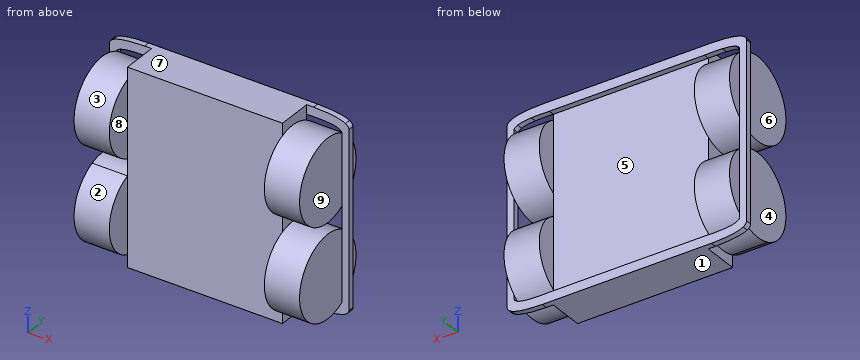
Autodesk Inventor part; units mm, degrees
ref_plane "YZ Plane" through (0, 0, 0) normal (1, 0, 0) x (0, 1, 0)
ref_plane "XZ Plane" through (0, 0, 0) normal (0, 1, 0) x (-1, 0, 0)
ref_plane "XY Plane" through (0, 0, 0) normal (0, 0, 1) x (1, 0, 0)
sketch "Эскиз1" plane through (0, 0, 0) normal (0, 1, 0) x (-1, 0, 0)
  line L0 (0, 0) -> (-132, 0)
  line L1 (-132, 0) -> (-132, -165.5)
  line L2 (-132, -165.5) -> (0, -165.5)
  line L3 (0, -165.5) -> (0, 0)
  line L4 (0, 0) -> (-132, 0)
  line L5 (-132, 0) -> (-132, -8)
  line L6 (-132, -8) -> (0, -8)
  line L7 (0, -8) -> (0, 0)
  line L8 (0, -165.5) -> (-132, -165.5)
  line L9 (-132, -165.5) -> (-132, -157.5)
  line L10 (-132, -157.5) -> (0, -157.5)
  line L11 (0, -157.5) -> (0, -165.5)
  line L12 (0, 0) -> (0, -43)
  line L13 (0, -43) -> (0, -8)
  line L14 (0, -8) -> (30, -8)
  line L15 (30, -8) -> (30, -78)
  line L16 (30, -78) -> (0, -78)
  line L17 (0, -78) -> (0, -8)
  line L18 (0, -157.5) -> (30, -157.5)
  line L19 (30, -157.5) -> (30, -87.5)
  line L20 (30, -87.5) -> (0, -87.5)
  line L21 (0, -87.5) -> (0, -157.5)
  line L22 (-132, -8) -> (-162, -8)
  line L23 (-162, -8) -> (-162, -78)
  line L24 (-162, -78) -> (-132, -78)
  line L25 (-132, -78) -> (-132, -8)
  line L26 (-132, -157.5) -> (-162, -157.5)
  line L27 (-162, -157.5) -> (-162, -87.5)
  line L28 (-162, -87.5) -> (-132, -87.5)
  line L29 (-132, -87.5) -> (-132, -157.5)
  dimension "d0" = 132
  dimension "d1" = 165.5
  dimension "d2" = 8
  dimension "d3" = 8
  dimension "d4" = 43
  dimension "d5" = 35
  dimension "d6" = 30
  dimension "d7" = 70
  dimension "d8" = 30
  dimension "d9" = 70
  dimension "d10" = 30
  dimension "d11" = 70
  dimension "d12" = 30
  dimension "d13" = 70
extrude "Выдавливание1" add sketch "Эскиз1" along normal blind 30 contours L3 L6 L1 L0 | L3 L10 L1 L6 | L10 L3 L2 L1
sketch "Эскиз2" plane through (132, 0, 0) normal (1, 0, 0) x (0, 0, -1)
  line L0 (0, 0) -> (0, 30)
  line L1 (165.5, 0) -> (165.5, 30)
  line L2 (165.5, 0) -> (0, 0)
  line L3 (0, 0) -> (43, 0)
  line L4 (43, 0) -> (43, 4.5763)
  line L5 (43, 4.5763) -> (43, 30)
  line L6 (43, 0) -> (43, 12.5)
  line L7 (165.5, 0) -> (122.5, 0)
  line L8 (122.5, 0) -> (122.5, 12.5)
  line L9 (122.5, 12.5) -> (43, 12.5)
  circle A0 centre (43, 12.5) radius 35
  circle A1 centre (122.5, 12.5) radius 35
  dimension "d24" = 43
  dimension "d25" = 12.5
  dimension "d26" = 43
  dimension "d27" = 70
  dimension "d28" = 70
extrude "Выдавливание2" add sketch "Эскиз2" along normal blind 30 contours A1 L2 | L2 L8 L9 A1 | L2 A1 L9 L8 | A0 L2 | L2 L4 L5 L9 A0 | L2 A0 L9 L5 L4
sketch "Эскиз3" plane through (0, 0, -165.5) normal (-1, 0, 0) x (0, 0, 1)
  circle A0 centre (122.5, 12.5) radius 35
  circle A1 centre (122.5, 12.5) radius 35
  arc A2 (10.3083, 0) -> (75.6917, 0) centre (43, 12.5) ccw
  circle A3 centre (43, 12.5) radius 35
  point P0 (165.5, 0)
  point P1 (122.5, 15)
  point P2 (43, 15)
  point P3 (75.6917, 0)
extrude "Выдавливание3" add sketch "Эскиз3" along normal blind 30
sketch "Эскиз4" plane through (0, 30, 0) normal (0, 1, 0) x (1, 0, 0)
  line L0 (-30, 78) -> (-30, 8)
  line L1 (-36, 8) -> (-36, 0)
  line L2 (132, 165.5) -> (0, 165.5)
  line L3 (-36, 0) -> (0, 0)
  line L4 (0, 0) -> (0, 165.5)
  line L5 (0, 165.5) -> (-36, 165.5)
  line L6 (-36, 165.5) -> (-36, 0)
  line L7 (132, 152.8109) -> (132, 165.5)
  line L8 (132, 165.5) -> (168, 165.5)
  line L9 (168, 165.5) -> (168, 0)
  line L10 (168, 0) -> (132, 0)
  line L11 (132, 0) -> (132, 165.5)
  line L12 (0, 8) -> (-30, 8)
  line L13 (-30, 157.5) -> (-30, 87.5)
  line L14 (0, 8) -> (-30, 8)
  line L15 (-30, 8) -> (-30, 157.5)
  line L16 (-30, 157.5) -> (0, 157.5)
  line L17 (0, 157.5) -> (0, 8)
  line L18 (162, 8) -> (162, 78)
  line L19 (132, 157.5) -> (162, 157.5)
  line L20 (162, 157.5) -> (162, 8)
  line L21 (162, 8) -> (132, 8)
  line L22 (132, 8) -> (132, 157.5)
  line L23 (168, 0) -> (-36, 0)
  line L24 (-36, 0) -> (-36, 165.5)
  line L25 (-36, 165.5) -> (168, 165.5)
  line L26 (168, 165.5) -> (168, 0)
  line L27 (0, 157.5) -> (132, 157.5)
  line L28 (132, 157.5) -> (132, 165.5)
  line L29 (132, 165.5) -> (0, 165.5)
  line L30 (0, 165.5) -> (0, 157.5)
  line L31 (0, 8) -> (0, 12.6891)
  line L32 (132, 0) -> (0, 0)
  line L33 (0, 0) -> (0, 8)
  line L34 (0, 8) -> (132, 8)
  line L35 (132, 8) -> (132, 0)
  line L36 (168, 165.5) -> (165, 165.5)
  line L37 (165, 165.5) -> (165, 161.5)
  line L38 (165, 161.5) -> (168, 161.5)
  line L39 (168, 161.5) -> (168, 165.5)
  line L40 (168, 0) -> (165, 0)
  line L41 (165, 0) -> (165, 4)
  line L42 (165, 4) -> (168, 4)
  line L43 (168, 4) -> (168, 0)
  line L44 (-36, 0) -> (-33, 0)
  line L45 (-33, 0) -> (-33, 4)
  line L46 (-33, 4) -> (-36, 4)
  line L47 (-36, 4) -> (-36, 0)
  line L48 (-36, 165.5) -> (-33, 165.5)
  line L49 (-33, 165.5) -> (-33, 161.5)
  line L50 (-33, 161.5) -> (-36, 161.5)
  line L51 (-36, 161.5) -> (-36, 165.5)
  line L52 (0, 165.5) -> (0, 155.1917)
  spline S0 degree 2 poles (0, 165.5) (-35.5316, 165.8812) (-36, 157.5) knots 0 0 0 1 1 1
  spline S1 degree 2 poles (132, 165.5) (167.5316, 165.8812) (168, 157.5) knots 0 0 0 1 1 1
  spline S2 degree 2 poles (132, 0) (167.5316, -0.3812) (168, 8) knots 0 0 0 1 1 1
  line L53 (0, 0) -> (132, 0)
  spline S3 degree 2 poles (0, 0) (-35.5316, -0.3812) (-36, 8) knots 0 0 0 1 1 1
  line L54 (-30, 8) -> (-27, 8)
  line L55 (-27, 8) -> (-27, 10)
  line L56 (-27, 10) -> (-30, 10)
  line L57 (-30, 10) -> (-30, 8)
  spline S4 degree 2 poles (0, 8) (-28.3192, 6.9002) (-30, 12.6891) knots 0 0 0 1 1 1
  line L58 (162, 8) -> (159, 8)
  line L59 (159, 8) -> (159, 10)
  line L60 (159, 10) -> (162, 10)
  line L61 (162, 10) -> (162, 8)
  line L62 (162, 157.5) -> (159, 157.5)
  line L63 (159, 157.5) -> (159, 155.5)
  line L64 (159, 155.5) -> (162, 155.5)
  line L65 (162, 155.5) -> (162, 157.5)
  line L66 (-30, 157.5) -> (-27, 157.5)
  line L67 (-27, 157.5) -> (-27, 155.5)
  line L68 (-27, 155.5) -> (-30, 155.5)
  line L69 (-30, 155.5) -> (-30, 157.5)
  spline S5 degree 2 poles (-30, 152.8109) (-28.3192, 158.5998) (0, 157.5) knots 0 0 0 1 1 1
  line L70 (162, 87.5) -> (162, 157.5)
  spline S6 degree 2 poles (132, 157.5) (160.3192, 158.5998) (162, 152.8109) knots 0 0 0 1 1 1
  spline S7 degree 2 poles (132, 8) (160.3192, 6.9002) (162, 12.6891) knots 0 0 0 1 1 1
  point P0 (0, 10.3083)
  point P1 (162, 152.8109)
  point P2 (137.9176, 0)
  point P3 (168, 8)
  point P4 (168, 157.5)
  point P5 (137.9176, 165.5)
  point P6 (-5.9176, 165.5)
  point P7 (-36, 157.5)
  point P8 (-5.9176, 0)
  point P9 (-30, 12.6891)
  point P10 (-30, 152.8109)
  dimension "d30" = 36
  dimension "d31" = 3
  dimension "d32" = 3
  dimension "d33" = 3
  dimension "d34" = 2
  dimension "d35" = 3
  dimension "d36" = 2
  dimension "d37" = 3
  dimension "d38" = 2
extrude "Выдавливание4" add sketch "Эскиз4" along normal blind 5 contours L0 L12 S4 L4 L3 S3 L6 S0 L5 S5 L16 L13 L15 | S4 L56 L0 | L56 L55 L12 L0 | S4 L12 L55 | L13 L68 S5 | L13 L16 L67 L68 | L67 L16 S5 | L34 L11 L23 L4 | S7 L21 L18 L20 L19 S6 L7 L8 S1 L9 S2 L10 L11 | L4 L2 L7 L27 | S7 L59 L21 | L59 L60 L18 L21 | S7 L18 L60 | L19 L63 S6 | L19 L20 L64 L63 | L64 L20 S6
sketch "Эскиз6" plane through (0, 30, 0) normal (0, 1, 0) x (1, 0, 0)
  line L0 (168, 8) -> (168, 157.5)
  line L1 (-36, 157.5) -> (-36, 8)
  line L2 (162, 16.1905) -> (162, 69.8095)
  line L3 (-30, 69.8095) -> (-30, 16.1905)
  line L4 (132, 12.6891) -> (132, 73.3109)
  line L5 (0, 73.3109) -> (0, 12.6891)
  line L6 (187.3576, 0) -> (377.3576, 0)
  line L7 (377.3576, 0) -> (377.3576, 165.5)
  line L8 (377.3576, 165.5) -> (187.3576, 165.5)
  line L9 (187.3576, 165.5) -> (187.3576, 0)
  point P0 (0, 0)
  dimension "d41" = 204
  dimension "d42" = 192
  dimension "d43" = 132
  dimension "d44" = 190
  dimension "d45" = 165.5
Part model, mm, in its own coordinate system. Face numbers are marked on the shaded views. A direction names the side the tool comes from. Coordinates: 2 decimals unless noted, no trailing zeros. Loops run counter-clockwise (first coordinate to the right, second up) from the corner with the lowest first, then second, coordinate; pieces in that order, holes last. Notation, with made-up numbers: (13, -32) - (58, -32) arc R27 cw to (58, -16) - close; hole circle Ø8 at (-8.75, 47.25). An arc over 180 degrees is marked (long way). Write item = value, one per line. Start each with the question number.
Item 1: 3-axis set-ups, long thin cutter, end or side, ignore diameter. For the marked faces 5, 6, 7, 8 and 9: which of +Z, -Z, +X, -X, +Y, -Y reach the whole face in a straight line?
Item 2: Flat gauge pins, fed straight in: pin 1 Ø10 at (y, z) = (43, -37.5) entering from -X; pin 2 Ø12 at (y, z) = (38.5, -71.5) entering from +X; pin 3 Ø24.5 at (y, z) = (-8.5, -116.5) entering from +X; pin 4 Ø8 at (x, z) = (122.5, -85) entering from -Y. Where does each tip first touch, or does it go through?
Item 3: Cut at D-D, the plane x = 142. State how many separate pieces and enclosed holes the cut face has, and give its area (3 significant figures).
Item 4: Cut at C-C, the plane z = -43. Give the cut face in (x, y).
Item 5: Wall check: L1, parallel to X at y = -10.5, z = -102.5; L2, parallel to Y at x = 122.5, z = -27; L3, parallel to X at y = 10, z = -22. Give the ranges that are in metal, low to high. Write a range as from..to.
Item 6: Mould opens along Z. For the marked faces 1, 2, 3 and 4 say: released by +Z, released by -Z, zero draft, split by the parting line, or undercut.
Item 7: Cut at B-B, the plane x = 96.5. Give the cut face in (y, z).
Item 8: Cut at A-A, the plane y = 12.5. Give the cut face in (x, z).
The answers:
q1.face_5 = +Y
q1.face_6 = +Z, -Z, -X, -Y
q1.face_7 = +Z, +X, -X, +Y, -Y
q1.face_8 = +Z, -Z, -Y
q1.face_9 = +Z, -Z, +X, -Y
q2.pin_1 = -30
q2.pin_2 = 168
q2.pin_3 = 162
q2.pin_4 = 0
q3.separate_pieces = 4
q3.enclosed_holes = 0
q3.area = 7,770 mm2
q4.outline = (-36, 30) - (-30, 30) - (-30, -22.5) - (0, -22.5) - (0, 0) - (132, 0) - (132, -22.5) - (162, -22.5) - (162, 30) - (168, 30) - (168, 35) - (162, 35) - (162, 47.5) - (132, 47.5) - (132, 30) - (0, 30) - (0, 47.5) - (-30, 47.5) - (-30, 35) - (-36, 35) - close
q5.L1 = -30..0, 132..162
q5.L2 = 0..30
q5.L3 = -30..162
q6.face_1 = released by -Z
q6.face_2 = undercut
q6.face_3 = undercut
q6.face_4 = zero draft
q7.outline = (0, -165.5) - (35, -165.5) - (35, -157.5) - (30, -157.5) - (30, -8) - (35, -8) - (35, 0) - (0, 0) - close
q8.outline = (-30, -157.5) - (0, -157.5) - (0, -165.5) - (132, -165.5) - (132, -157.5) - (162, -157.5) - (162, -87.5) - (132, -87.5) - (132, -78) - (162, -78) - (162, -8) - (132, -8) - (132, 0) - (0, 0) - (0, -8) - (-30, -8) - (-30, -78) - (0, -78) - (0, -87.5) - (-30, -87.5) - close
